Autodesk Inventor part; units mm, degrees
ref_plane "YZ Plane" through (0, 0, 0) normal (1, 0, 0) x (0, 1, 0)
ref_plane "XZ Plane" through (0, 0, 0) normal (0, 1, 0) x (-1, 0, 0)
ref_plane "XY Plane" through (0, 0, 0) normal (0, 0, 1) x (1, 0, 0)
sketch "Sketch1" plane through (0, 0, 0) normal (0, 1, 0) x (-1, 0, 0)
  line L0 (0, 0) -> (34, 0)
  line L1 (34, 0) -> (34, -11.1)
  line L2 (34, -11.1) -> (0, -11.1)
  line L3 (0, -11.1) -> (0, 0)
  dimension "d0" = 34
  dimension "d1" = 11.1
extrude "Extrusion1" add sketch "Sketch1" along normal blind 3.5
sketch "Sketch2" plane through (0, 3.5, 0) normal (0, 1, 0) x (1, 0, 0)
  line L0 (-32.8, 0.5) -> (-1.2, 0.5)
  line L1 (-1.2, 0.5) -> (-1.2, 10.6)
  line L2 (-1.2, 10.6) -> (-32.8, 10.6)
  line L3 (-32.8, 10.6) -> (-32.8, 0.5)
  line L4 (-34, 11.1) -> (-34, 0)
  line L5 (0, 0) -> (0, 11.1)
  line L6 (0, 11.1) -> (-34, 11.1)
  line L7 (-34, 0) -> (0, 0)
  dimension "d4" = 1.2
  dimension "d5" = 1.2
  dimension "d6" = 0.5
  dimension "d7" = 0.5
extrude "Extrusion2" cut sketch "Sketch2" against normal blind 1
sketch "Sketch3" plane through (0, 0, 0) normal (0, -1, 0) x (1, 0, 0)
  line L0 (-0.55, -10.5) -> (-33.45, -10.5)
  line L1 (-33.45, -10.5) -> (-33.45, -0.6)
  line L2 (-33.45, -0.6) -> (-0.55, -0.6)
  line L3 (-0.55, -0.6) -> (-0.55, -10.5)
  line L4 (-0.55, -10.5) -> (-33.45, -0.6) construction
  line L5 (-33.45, -10.5) -> (-0.55, -0.6) construction
  line L6 (-17, -5.55) -> (-17, -7.3465)
  line L7 (-17, -7.3465) -> (-17, -5.55)
  line L8 (-22.3316, -5.55) -> (-22.3865, -5.55)
  line L9 (-22.3865, -5.55) -> (-17, -5.55)
  line L10 (-34, -11.1) -> (-34, 0)
  line L11 (0, -11.1) -> (-34, -11.1)
  line L12 (0, -11.1) -> (-34, -11.1)
  line L13 (0, 0) -> (0, -11.1)
  line L14 (-34, 0) -> (0, 0)
  line L15 (-34, -11.1) -> (-34, 0)
  point P0 (-34, -5.55)
  point P1 (-17, -11.1)
  dimension "d10" = 32.9
  dimension "d11" = 9.9
extrude "Extrusion3" cut sketch "Sketch3" against normal blind 0.25
fillet "Fillet1" radius 2 4 edges at (-33.45, 0.125, -10.5) (-33.45, 0.125, -0.6) (-0.55, 0.125, -0.6) (-0.55, 0.125, -10.5)
fillet "Fillet2" radius 0.5 4 edges at (-34, 1.375, 0) (-34, 1.375, -11.1) (0, 1.375, 0) (0, 1.375, -11.1)
chamfer "Chamfer1" distance 2 angle 45 4 edges at (-1.2, 3, -0.5) (-1.2, 3, -10.6) (-32.8, 3, -0.5) (-32.8, 3, -10.6)
equation "\"d5\" = d4"
equation "\"d7\" = d6"
properties part number "Speka" material "Acetal Resin, Black"
Design review of the part built by this model. Coordinates are the model's own, in mm. A direction names the side the tool comes from. Give positions to 0.01 mm unless a question says otherwise; leave off trailing zeros. Loops run counter-clockwise (first coordinate to the right, second up) from the corner with the lowest first, then second, coordinate; pieces in that order, holes last. Notation, with made-up numbers: (-37.75, -3) - (-8.75, -3) arc R21 cw to (-8.75, 21) - close; hole circle Ø5 at (27.25, 69). An arc over 180 degrees is marked (long way). Write item = value, one per line.
1) Clearance check with flat-ended pins moving along their axes: pin 1 Ø0.8 at (y, z) = (3, -6.5) entering from -X; pin 2 Ø0.8 at (x, y) = (-12.5, 3) entering from -Z. State where each tip first meets the part, or that it passes through.
Result sheet:
pin_1 = -32.8
pin_2 = -10.6
2) To check wall thickness, follow line 1 (X direction, y = 3.15, z = -8.5); line 2 (Z direction, x = -22, y = 2.7); line 3 (Z direction, x = -2.5, y = 0.2). State the ranges of each line that lie inside material, in increasing order.
Result sheet:
line_1 = -32.8 to -1.2
line_2 = -10.6 to -0.5
line_3 = -10.5 to -0.6
3) Take a section at B-B on z = -5.5. State the section outline as (x, y) points, and give its area (3 significant figures).
Result sheet:
outline = (-34, 0.25) - (-33.45, 0.25) - (-33.45, 0) - (-0.55, 0) - (-0.55, 0.25) - (0, 0.25) - (0, 2.5) - (-1.2, 2.5) - (-1.2, 3.5) - (-32.8, 3.5) - (-32.8, 2.5) - (-34, 2.5) - close
area = 116 mm2
4) Tool access review of faces 1 (the face through (-31.8, 3, -1.5)), 2 (the face through (-2.2, 3, -9.6)), 3 (the face through (-1.2, 3, -6)): name each direction out of +Z, -Z, +X, -X, +Y, -Y from which nothing blocks a thin tool from reaching the whole face with its end or side.
Result sheet:
face_1 = +Z, -X, +Y
face_2 = -Z, +X, +Y
face_3 = +Z, -Z, +X, +Y
5) Take a section at A-A on x = -17. State the section outline as (y, z) points, and give its area (4 significant figures).
Result sheet:
outline = (0, -10.5) - (0.25, -10.5) - (0.25, -11.1) - (2.5, -11.1) - (2.5, -10.6) - (3.5, -10.6) - (3.5, -0.5) - (2.5, -0.5) - (2.5, 0) - (0.25, 0) - (0.25, -0.6) - (0, -0.6) - close
area = 37.55 mm2
6) Take a section at C-C on y = 3. State the section outline as (x, z) points.
Result sheet:
outline = (-32.8, -8.6) - (-30.8, -10.6) - (-3.2, -10.6) - (-1.2, -8.6) - (-1.2, -2.5) - (-3.2, -0.5) - (-30.8, -0.5) - (-32.8, -2.5) - close
